Source: CAD feature listing. Evaluate the final solid. Frame: model axes, mm. Face numbers are marked on the shaded views. A direction names the side the tool comes from. Round coordinates to 2 decimals unless told otherwise and drop trailing zeros. Order: outer loops, then holes, each group sorted by start corner. A loop starts at its lowest first (then second) coordinate and runs counter-clockwise, first axis right, second up. Notation, with made-up numbers: M -7.75,55 L 20.25,55 A21 cw 20.25,83 Z; hole C -17,26.25 d3. An arc over 180 degrees is marked long. Answer as CSV lines item,"result". Start each with the question number.
Item 1: Set-up query: the marked faces 4 and 5. Return all of +Z, -Z, +X, -X, +Y, -Y with unobstructed straight access to the full face (end or side cutting, diameter ignored); none if empty.
Item 2: Section query B-B on x = 12.7. Return the cut outline in (y, z).
Item 3: Line query: line 1 (X direction, y = 1, z = 19); line 2 (Z direction, x = 12.7, y = 1.5); line 3 (Z direction, x = 1, y = 25). Output: solid intervals per line, ascending. Write a range as [from, to].
Item 4: First-contact query: P1, Ø4, axis at x = 28.5, z = -3.5, coming from the +Y side; P2, Ø8, axis at y = 38.5, z = -11, coming from the +X side; P3, Ø23.5, axis at y = 25.4, z = -6.35, coming from the -X side. Flat tips, straight axial feed; report the tip coordinate or a pass-through.
Item 5: Section query D-D on z = 19.05. Return the cut outline in (x, y) (3 decimals).
Item 6: Pull-direction query (Y, two-part tool) for the marked faces 1, 2 and 3; classes: +Y half, -Y half, draft (parallel to the pull), parting line (faces both ways), or undercut.
Item 7: Section query C-C on z = -6.35. Return the cut outline in (x, y) (3 decimals), plus the area to 3 significant figures.
Item 8: Section query A-A on y = 25.4. Return the cut outline in (x, z).
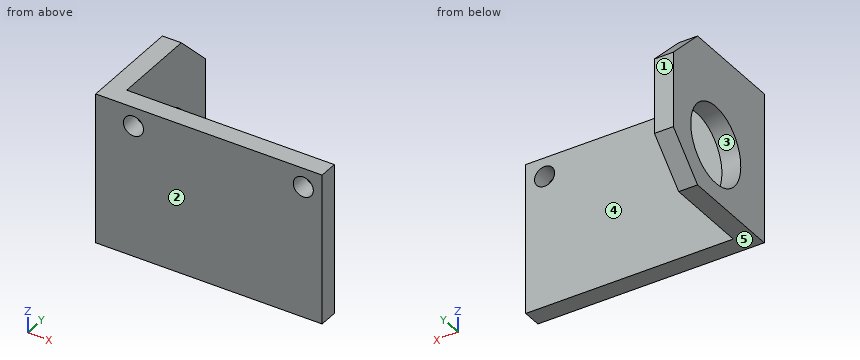
from build123d import *

# Parameters (mm, degrees)
BOSS_EXTRUDE1_DEPTH     = 25.4
F_1_4_CLEARANCE_HOLE1_D = 6.7564
F_1_CLEARANCE_HOLE1_D   = 26.19248
CHAMFER1_SIZE           = 12.7


with BuildPart() as part:
    # Sketch1 → Boss-Extrude1 (new, symmetric)
    with BuildSketch(Plane.XY):
        Polygon((0, 0), (76.2, 0), (76.2, 6.35), (6.35, 6.35), (6.35, 47.625), (0, 47.625), align=None)
    extrude(amount=BOSS_EXTRUDE1_DEPTH, both=True)

    # 1/4 Clearance Hole1 (through all)
    with Locations(Plane(origin=(0, 0, 0), x_dir=(-1, 0, 0), z_dir=(0, -1, 0))):
        with Locations((-12.7, -19.05), (-69.85, -19.05)):
            Hole(F_1_4_CLEARANCE_HOLE1_D / 2)

    # 1 Clearance Hole1 (through all)
    with Locations(Plane.ZY):
        with Locations((-6.35, 25.4)):
            Hole(F_1_CLEARANCE_HOLE1_D / 2)

    # Chamfer1
    chamfer1_edges = [part.edges().sort_by_distance(p)[0] for p in [
        (3.175, 47.625, 25.4),
        (3.175, 47.625, -25.4),
    ]]
    chamfer(chamfer1_edges, length=CHAMFER1_SIZE)


solid = part.part
Results:
1,face 4,"+Z, -Z, +X, +Y"
1,face 5,"-Z, +X, -X, +Y, -Y"
2,outline,"M 0,-25.4 L 6.35,-25.4 L 6.35,15.67 L 0,15.67 Z; M 0,22.43 L 6.35,22.43 L 6.35,25.4 L 0,25.4 Z"
3,line 1,"[0, 9.32], [16.08, 66.47], [73.23, 76.2]"
3,line 2,"[-25.4, 15.67], [22.43, 25.4]"
3,line 3,"[-25.4, -19.44], [6.74, 25.4]"
4,P1,"y = 6.35"
4,P2,"x = 6.35"
4,P3,"through"
5,outline,"M 0,0 L 9.322,0 L 9.322,6.35 L 6.35,6.35 L 6.35,41.275 L 0,41.275 Z; M 16.078,0 L 66.472,0 L 66.472,6.35 L 16.078,6.35 Z; M 73.228,0 L 76.2,0 L 76.2,6.35 L 73.228,6.35 Z"
6,face 1,"+Y half"
6,face 2,"-Y half"
6,face 3,"undercut"
7,outline,"M 0,0 L 76.2,0 L 76.2,6.35 L 6.35,6.35 L 6.35,12.304 L 0,12.304 Z; M 0,38.496 L 6.35,38.496 L 6.35,47.625 L 0,47.625 Z"
7,area,"580 mm^2"
8,outline,"M 0,-25.4 L 6.35,-25.4 L 6.35,-19.45 L 0,-19.45 Z; M 0,6.75 L 6.35,6.75 L 6.35,25.4 L 0,25.4 Z"
